The model under review builds one solid part; all positions refer to its coordinate system, in mm. A direction names the side the tool comes from. Round coordinates to 2 decimals unless told otherwise and drop trailing zeros. Write each loop counter-clockwise with the first axis right and the second up, starting at its lowest first coordinate (ties: lowest second). Pieces come first, ordered by that corner, then holes. Notation, with made-up numbers: (-5.5, 17) -> (13.5, 17) arc R15 ccw to (13.5, 29) -> close; hole circle Ø6 at (14.25, 80.25). An arc over 180 degrees is marked (long way). Return JSON: item names as keys, results as strings. Group by question number.
1. For line 1 along Z through (x, y) = (-8.75, -1.85); line 2 along X through (y, z) = (2.7, 0) (3 decimals); line 3 along X through (y, z) = (-2.2, -9), list the stretches that pass through material, from the lowest coordinate up. Write a range as from..to.
2. Take a section at B-B, the plane z = 3.75. Write out the cut boundary in (x, y), then the cut area to 3 significant figures.
3. Take a section at D-D, the plane x = -2. Write out the cut boundary in (y, z), then the cut area to 3 significant figures.
4. Take a section at C-C, the plane x = 6. Write out the cut boundary in (y, z), then the cut area to 3 significant figures.
5. Mouldability with a two-part tool opening along X and no side actions: class faces 1 (the flat face through (3, -1.3, 9.8)), 2 (the cylindrical face through (0, -1, 16)), 3 (the flat face through (-9.93, -1.33, 2.26)) as pulls with the +X half, pulls with the -X half, needs draft (parallel to the pull), parting line crosses it, or undercut.
6. Clearance check with flat-ended pins moving along their axes: P1, Ø1.2, axis at x = 9.09, z = 5.25, coming from the -Y side; P2, Ø1, axis at x = 1, y = 2, coming from the -Z side; P3, Ø3, axis at x = -9.09, z = -5.25, coming from the +Y side; P4, Ø2, axis at y = -1, z = 0, coming from the -X side. State where each tip first meets the part, or that it passes through.
7. Tool access review of faces 4 (the flat face through (-10.017, -1.331, -2.325)), 5 (the flat face through (6.92, -1.33, 7.47)), 6 (the flat face through (-3, -1.3, -9.8)), 7 (the cylindrical face through (-8.117, -1.331, -5.033)): name each direction out of +Z, -Z, +X, -X, +Y, -Y from which nothing blocks a thin tool from reaching the whole face with its end or side.
8. Take a section at A-A, the plane z = 10.5. Write out the cut boundary in (x, y), then the cut area to 3 significant figures.
from build123d import *

# Parameters (mm, degrees)
SKETCH1_R                    = 4.325
BOSS_EXTRUDE1_DEPTH          = 3
SKETCH2_R                    = 2.5
BOSS_EXTRUDE2_DEPTH          = 2.7
SKETCH3_R                    = 1
CUT_EXTRUDE1_DEPTH           = 2.7
LPATTERN1_COUNT              = 3
LPATTERN1_PITCH              = 3
CIRPATTERN1_COUNT            = 6
CIRPATTERN1_COPY_1_SKETCH_R  = 1
CIRPATTERN1_COPY_1_DEPTH     = 2.7
CIRPATTERN1_COPY_2_SKETCH_R  = 1
CIRPATTERN1_COPY_2_DEPTH     = 2.7
CIRPATTERN1_COPY_3_SKETCH_R  = 1
CIRPATTERN1_COPY_3_DEPTH     = 2.7
CIRPATTERN1_COPY_4_SKETCH_R  = 1
CIRPATTERN1_COPY_4_DEPTH     = 2.7
CIRPATTERN1_COPY_5_SKETCH_R  = 1
CIRPATTERN1_COPY_5_DEPTH     = 2.7
CIRPATTERN1_COPY_6_SKETCH_R  = 1
CIRPATTERN1_COPY_6_DEPTH     = 2.7
CIRPATTERN1_COPY_7_SKETCH_R  = 1
CIRPATTERN1_COPY_7_DEPTH     = 2.7
CIRPATTERN1_COPY_8_SKETCH_R  = 1
CIRPATTERN1_COPY_8_DEPTH     = 2.7
CIRPATTERN1_COPY_9_SKETCH_R  = 1
CIRPATTERN1_COPY_9_DEPTH     = 2.7
CIRPATTERN1_COPY_10_SKETCH_R = 1
CIRPATTERN1_COPY_10_DEPTH    = 2.7
SKETCH6_R                    = 2.85
CUT_EXTRUDE2_DEPTH           = 3.4
CUT_EXTRUDE3_REACH           = 23.655
SKETCH7_R                    = 1.5


with BuildPart() as part:
    # Sketch1 → Boss-Extrude1 (new body)
    with BuildSketch(Plane(origin=(0, 0, 0), x_dir=(1, 0, 0), z_dir=(0, 1, 0))):
        with Locations(Location((0, 0, 0), (0, 0, 270))):
            Circle(SKETCH1_R)
    extrude(amount=BOSS_EXTRUDE1_DEPTH)

    # Sketch2 → Boss-Extrude2 (add)
    with BuildSketch(Plane(origin=(0, 0, 0), x_dir=(1, 0, 0), z_dir=(0, 1, 0))):
        with Locations((0, 13.5)):
            Circle(SKETCH2_R)
        Polygon((-4.325, 0), (4.325, 0), (2.5, 13.5), (-2.5, 13.5), align=None)
    boss_extrude2 = extrude(amount=-BOSS_EXTRUDE2_DEPTH)

    # Sketch3 → Cut-Extrude1 (cut)
    with BuildSketch(Plane(origin=(0, 0, 0), x_dir=(1, 0, 0), z_dir=(0, 1, 0))):
        with Locations(Location((0, 13.5, 0), (0, 0, 270))):
            Circle(SKETCH3_R)
    cut_extrude1 = extrude(amount=-CUT_EXTRUDE1_DEPTH, mode=Mode.SUBTRACT)

    # LPattern1: Cut-Extrude1 ×3
    with Locations(*[(0, 0, i * LPATTERN1_PITCH) for i in range(1, LPATTERN1_COUNT)]):
        add(cut_extrude1, mode=Mode.SUBTRACT)

    # CirPattern1: Boss-Extrude2, Cut-Extrude1 ×6 about axis
    cirpattern1_axis = Axis((0, 0, 0), (0, 1, 0))
    add([boss_extrude2.rotate(cirpattern1_axis, i * 360 / CIRPATTERN1_COUNT) for i in range(1, CIRPATTERN1_COUNT)])
    add([cut_extrude1.rotate(cirpattern1_axis, i * 360 / CIRPATTERN1_COUNT) for i in range(1, CIRPATTERN1_COUNT)], mode=Mode.SUBTRACT)

    # CirPattern1 copy 1 sketch → CirPattern1 copy 1 (cut)
    with BuildSketch(Plane(origin=(2.598076211, 0, 1.5), x_dir=(0.5000000000000001, 0, -0.8660254037844386), z_dir=(0, 1, 0))):
        with Locations(Location((0, 13.5, 0), (0, 0, 270))):
            Circle(CIRPATTERN1_COPY_1_SKETCH_R)
    extrude(amount=-CIRPATTERN1_COPY_1_DEPTH, mode=Mode.SUBTRACT)

    # CirPattern1 copy 2 sketch → CirPattern1 copy 2 (cut)
    with BuildSketch(Plane(origin=(2.598076211, 0, -1.5), x_dir=(-0.4999999999999998, 0, -0.8660254037844387), z_dir=(0, 1, 0))):
        with Locations(Location((0, 13.5, 0), (0, 0, 270))):
            Circle(CIRPATTERN1_COPY_2_SKETCH_R)
    extrude(amount=-CIRPATTERN1_COPY_2_DEPTH, mode=Mode.SUBTRACT)

    # CirPattern1 copy 3 sketch → CirPattern1 copy 3 (cut)
    with BuildSketch(Plane(origin=(0, 0, -3), x_dir=(-1, 0, 0), z_dir=(0, 1, 0))):
        with Locations(Location((0, 13.5, 0), (0, 0, 270))):
            Circle(CIRPATTERN1_COPY_3_SKETCH_R)
    extrude(amount=-CIRPATTERN1_COPY_3_DEPTH, mode=Mode.SUBTRACT)

    # CirPattern1 copy 4 sketch → CirPattern1 copy 4 (cut)
    with BuildSketch(Plane(origin=(-2.598076211, 0, -1.5), x_dir=(-0.5000000000000004, 0, 0.8660254037844384), z_dir=(0, 1, 0))):
        with Locations(Location((0, 13.5, 0), (0, 0, 270))):
            Circle(CIRPATTERN1_COPY_4_SKETCH_R)
    extrude(amount=-CIRPATTERN1_COPY_4_DEPTH, mode=Mode.SUBTRACT)

    # CirPattern1 copy 5 sketch → CirPattern1 copy 5 (cut)
    with BuildSketch(Plane(origin=(-2.598076211, 0, 1.5), x_dir=(0.5000000000000001, 0, 0.8660254037844386), z_dir=(0, 1, 0))):
        with Locations(Location((0, 13.5, 0), (0, 0, 270))):
            Circle(CIRPATTERN1_COPY_5_SKETCH_R)
    extrude(amount=-CIRPATTERN1_COPY_5_DEPTH, mode=Mode.SUBTRACT)

    # CirPattern1 copy 6 sketch → CirPattern1 copy 6 (cut)
    with BuildSketch(Plane(origin=(5.196152423, 0, 3), x_dir=(0.5000000000000001, 0, -0.8660254037844386), z_dir=(0, 1, 0))):
        with Locations(Location((0, 13.5, 0), (0, 0, 270))):
            Circle(CIRPATTERN1_COPY_6_SKETCH_R)
    extrude(amount=-CIRPATTERN1_COPY_6_DEPTH, mode=Mode.SUBTRACT)

    # CirPattern1 copy 7 sketch → CirPattern1 copy 7 (cut)
    with BuildSketch(Plane(origin=(5.196152423, 0, -3), x_dir=(-0.4999999999999998, 0, -0.8660254037844387), z_dir=(0, 1, 0))):
        with Locations(Location((0, 13.5, 0), (0, 0, 270))):
            Circle(CIRPATTERN1_COPY_7_SKETCH_R)
    extrude(amount=-CIRPATTERN1_COPY_7_DEPTH, mode=Mode.SUBTRACT)

    # CirPattern1 copy 8 sketch → CirPattern1 copy 8 (cut)
    with BuildSketch(Plane(origin=(0, 0, -6), x_dir=(-1, 0, 0), z_dir=(0, 1, 0))):
        with Locations(Location((0, 13.5, 0), (0, 0, 270))):
            Circle(CIRPATTERN1_COPY_8_SKETCH_R)
    extrude(amount=-CIRPATTERN1_COPY_8_DEPTH, mode=Mode.SUBTRACT)

    # CirPattern1 copy 9 sketch → CirPattern1 copy 9 (cut)
    with BuildSketch(Plane(origin=(-5.196152423, 0, -3), x_dir=(-0.5000000000000004, 0, 0.8660254037844384), z_dir=(0, 1, 0))):
        with Locations(Location((0, 13.5, 0), (0, 0, 270))):
            Circle(CIRPATTERN1_COPY_9_SKETCH_R)
    extrude(amount=-CIRPATTERN1_COPY_9_DEPTH, mode=Mode.SUBTRACT)

    # CirPattern1 copy 10 sketch → CirPattern1 copy 10 (cut)
    with BuildSketch(Plane(origin=(-5.196152423, 0, 3), x_dir=(0.5000000000000001, 0, 0.8660254037844386), z_dir=(0, 1, 0))):
        with Locations(Location((0, 13.5, 0), (0, 0, 270))):
            Circle(CIRPATTERN1_COPY_10_SKETCH_R)
    extrude(amount=-CIRPATTERN1_COPY_10_DEPTH, mode=Mode.SUBTRACT)

    # Sketch6 → Cut-Extrude2 (cut)
    with BuildSketch(Plane(origin=(0, 3, 0), x_dir=(1, 0, 0), z_dir=(0, 1, 0))):
        with Locations(Location((0, 0, 0), (0, 0, 270))):
            Circle(SKETCH6_R)
    extrude(amount=-CUT_EXTRUDE2_DEPTH, mode=Mode.SUBTRACT)

    # Sketch7 → Cut-Extrude3 (cut, up to next)
    with BuildSketch(Plane(origin=(0, -0.4, 0), x_dir=(1, 0, 0), z_dir=(0, 1, 0)), mode=Mode.PRIVATE) as cut_extrude3_sk1:
        with Locations(Location((0, 0, 0), (0, 0, 270))):
            Circle(SKETCH7_R)
    cut_extrude3_tool1 = extrude(cut_extrude3_sk1.sketch, amount=-CUT_EXTRUDE3_REACH, mode=Mode.PRIVATE) & part.part
    add(cut_extrude3_tool1.solids().sort_by_distance((0, -0.4, 0))[0], mode=Mode.SUBTRACT)


solid = part.part
Output:
{
 "1": {"line 1": "z = -8.22..-6.19, -4.31..-1.35, 1.35..4.31, 6.19..8.22", "line 2": "x = -4.325..-2.85, 2.85..4.325", "line 3": "x = -12.78..-10.6, -3.11..3.11, 10.6..12.78"},
 "2": {"outline": "(-11.86, -2.7) -> (-7.5, -2.7) -> (-7.5, 0) -> (-11.86, 0) -> close; (-5.5, -2.7) -> (5.5, -2.7) -> (5.5, 0) -> (2.15, 0) -> (2.15, 3) -> (-2.15, 3) -> (-2.15, 0) -> (-5.5, 0) -> close; (7.5, -2.7) -> (11.86, -2.7) -> (11.86, 0) -> (7.5, 0) -> close", "area": "66.2 mm^2"},
 "3": {"outline": "(-2.7, -15) -> (0, -15) -> (0, -3.83) -> (3, -3.83) -> (3, -2.03) -> (-0.4, -2.03) -> (-0.4, 2.03) -> (3, 2.03) -> (3, 3.83) -> (0, 3.83) -> (0, 15) -> (-2.7, 15) -> close", "area": "90.2 mm^2"},
 "4": {"outline": "(-2.7, -7.09) -> (0, -7.09) -> (0, -4.62) -> (-2.7, -4.62) -> close; (-2.7, -2.88) -> (0, -2.88) -> (0, 2.88) -> (-2.7, 2.88) -> close; (-2.7, 4.62) -> (0, 4.62) -> (0, 7.09) -> (-2.7, 7.09) -> close", "area": "28.9 mm^2"},
 "5": {"face 1": "undercut", "face 2": "parting line crosses it", "face 3": "pulls with the -X half"},
 "6": {"P1": "passes through", "P2": "stops at z = -4.3", "P3": "stops at y = 0", "P4": "stops at x = -8.3"},
 "7": {"face 4": "-X, +Y, -Y", "face 5": "+Z, +Y, -Y", "face 6": "-Z, +Y, -Y", "face 7": "+Y, -Y"},
 "8": {"outline": "(-2.91, -2.7) -> (-1, -2.7) -> (-1, 0) -> (-2.91, 0) -> close; (1, -2.7) -> (2.91, -2.7) -> (2.91, 0) -> (1, 0) -> close", "area": "10.3 mm^2"}
}
